from build123d import *

# Parameters (mm, degrees)
F1_DEPTH = 19.05
F3_D     = 12.7
F5_D     = 12.7
F6_R     = 2.54


with BuildPart() as f1:
    # F0 (on Top) → F1 (new body)
    with BuildSketch(Plane.XY):
        Polygon((45.404016, 2.31187), (-1.694917, 2.31187), (-1.694917, 8.66187), (-35.984917, 8.66187), (-35.984917, 2.31187), (-7.148128, 2.31187), (-7.148128, -23.08813), (-35.984917, -23.08813), (-35.984917, -29.43813), (-1.694917, -29.43813), (-1.694917, -23.08813), (45.404016, -23.08813), (45.404016, -29.43813), (79.694016, -29.43813), (79.694016, -23.08813), (50.865016, -23.08813), (50.865016, 2.31187), (79.694016, 2.31187), (79.694016, 8.66187), (45.404016, 8.66187), align=None)
    extrude(amount=F1_DEPTH)

    # F3 (through all)
    with Locations(Plane.XZ.offset(29.43813)):
        with Locations((-26.459917, 9.525)):
            Hole(F3_D / 2)

    # F5 (through all)
    with Locations(Plane.XZ.offset(29.43813)):
        with Locations((70.169016, 9.525)):
            Hole(F5_D / 2)

    # F6
    f6_edges = [f1.edges().sort_by_distance(p)[0] for p in [
        (50.865016, -10.38813, 19.05),
        (50.865016, -10.38813, 0),
        (-7.148128, -10.38813, 19.05),
        (-7.148128, -10.38813, 0),
    ]]
    fillet(f6_edges, radius=F6_R)


solid = f1.part
CAD build for the part. Positions are in the model's coordinates, mm. A direction names the side the tool comes from. Round coordinates to 2 decimals unless told otherwise and drop trailing zeros. Write each loop counter-clockwise with the first axis right and the second up, starting at its lowest first coordinate (ties: lowest second). Pieces come first, ordered by that corner, then holes. Notation, with made-up numbers: (74.5, 3) -> (98.5, 3) arc R7 cw to (98.5, 10) -> close; hole circle Ø5 at (82, -2.75). An arc over 180 degrees is marked (long way). Answer as a JSON object with one key per item and string values.
(1) Which spindle directions (+Z, -Z, +X, -X, +Y, -Y) get a long thin tool onto all of the face, cutting with end or side? Do faces 4 (the face through (-6.38, -10.57, 0.72)), 5 (the face through (-7.148, -10, 9)), 6 (the face through (22, 2.312, 9)). Say none if no direction does.
Reported:
{"face 4": "-Z, -X", "face 5": "+Z, -Z, -X", "face 6": "+Z, -Z, +Y"}
(2) Probe probe 1 along Y at (x, z) = (65.5, 16); probe 2 along X at (y, z) = (4, 8.75); probe 3 along X at (y, z) = (5, 8.25). List the from-to ranges inside material, lowest first. Write a range as [from, to].
Reported:
{"probe 1": "y = [-29.44, -23.09], [2.31, 8.66]", "probe 2": "x = [-35.98, -32.76], [-20.16, -1.69], [45.4, 63.87], [76.47, 79.69]", "probe 3": "x = [-35.98, -32.68], [-20.24, -1.69], [45.4, 63.95], [76.39, 79.69]"}
(3) Band-saw the part on B-B, the plane z = 8.25. Count the separate pieces of the cut face and the enclosed holes in it, then the cut area to 3 significant figures.
Reported:
{"separate pieces": "5", "enclosed holes": "0", "area": "2,030 mm^2"}
(4) Band-saw the part on A-A, the plane y = -4. List the corners of the cut face in (x, z), then the cut area to 3 significant figures.
Reported:
{"outline": "(-7.15, 2.54) arc R2.54 ccw to (-4.61, 0) -> (48.33, 0) arc R2.54 ccw to (50.87, 2.54) -> (50.87, 16.51) arc R2.54 ccw to (48.33, 19.05) -> (-4.61, 19.05) arc R2.54 ccw to (-7.15, 16.51) -> close", "area": "1,100 mm^2"}
(5) Pin check, flat tips, straight feed: P1, Ø1, axis at x = 37.5, z = 11.5, coming from the -Y side; P2, Ø10, axis at x = 15, z = 2, coming from the +Y side; P3, Ø7, axis at y = -14.5, z = 13, coming from the -X side. Stop position of each tip, or through.
Reported:
{"P1": "stops at y = -23.09", "P2": "stops at y = 2.31", "P3": "stops at x = -7.15"}
(6) Two-plate mould, pull along Z, no slides. Class faces 1 (the face through (-6.38, -10.57, 18.33)), 2 (the face through (-20, -23.088, 7)), 3 (the face through (-29.39, 5.53, 3.89)): +Z half, -Z half, draft (parallel to the pull), parting line (faces both ways), or undercut.
Reported:
{"face 1": "+Z half", "face 2": "draft", "face 3": "undercut"}
(7) Band-saw the part on C-C, the plane x = 12. List the corners of the cut face in (y, z).
Reported:
{"outline": "(-23.09, 0) -> (2.31, 0) -> (2.31, 19.05) -> (-23.09, 19.05) -> close"}
